```python
from build123d import *

# Parameters (mm, degrees)
EXTRUDE_1_DEPTH          = 2.5
SKETCH_4_W               = 70.612
SKETCH_4_H               = 2
EXTRUDE_2_DEPTH          = 10
SKETCH_5_R               = 4.19
SKETCH_5_R_2             = 4.191
EXTRUDE_3_DEPTH          = 12.5
SKETCH_7_R               = 2.7083489
SKETCH_7_R_2             = 2.708349387
CUT_EXTRUDE_1_DEPTH      = 10.5
CUT_EXTRUDE_2_DEPTH      = 48.585689944
CUT_EXTRUDE_2_DEPTH_BACK = 48.585689944
SKETCH_8_R               = 1.65


with BuildPart() as part:
    # 草图3 → 凸台-拉伸1 (new body)
    with BuildSketch(Plane.XY):
        with BuildLine():
            Line((-36.295196216, 26.676238556), (32.166947784, 26.676238556))
            ThreePointArc((32.166947784, 26.676238556), (32.927036662, 26.361399434), (33.241875784, 25.601310556))
            Line((33.241875784, 25.601310556), (33.241875784, -11.394297444))
            Line((33.241875784, -11.394297444), (-37.370124216, -11.320561244))
            Line((-37.370124216, -11.320561244), (-37.370124216, 25.601297856))
            ThreePointArc((-37.370124216, 25.601297856), (-37.055289584, 26.361394944), (-36.295196216, 26.676238556))
        make_face()
    extrude(amount=-EXTRUDE_1_DEPTH)

    # 草图4 → 凸台-拉伸2 (add)
    with BuildSketch(Plane(origin=(0, 0, -2.5), x_dir=(-1, 0, 0), z_dir=(0, 0, -1))):
        with Locations((2.064124216, -10.394297444)):
            Rectangle(SKETCH_4_W, SKETCH_4_H)
    extrude(amount=EXTRUDE_2_DEPTH)

    # 草图5 → 凸台-拉伸3 (add)
    with BuildSketch(Plane.XY):
        with Locations((-7.906124216, -5.962761444)):
            Circle(SKETCH_5_R)
        with Locations((28.796875784, 22.485238556)):
            Circle(SKETCH_5_R_2)
    extrude(amount=-EXTRUDE_3_DEPTH)

    # 草图7 → 切除-拉伸1 (cut)
    with BuildSketch(Plane.XY):
        with Locations((-7.906124216, -5.962761444)):
            Circle(SKETCH_7_R)
        with Locations((28.796875784, 22.485238556)):
            Circle(SKETCH_7_R_2)
    extrude(amount=-CUT_EXTRUDE_1_DEPTH, mode=Mode.SUBTRACT)

    # 草图8 → 切除-拉伸2 (cut, two sides: drawn at the far end of the back side and taken through both)
    with BuildSketch(Plane(origin=(0, 0, -12.5), x_dir=(-1, 0, 0), z_dir=(0, 0, -1)).offset(-CUT_EXTRUDE_2_DEPTH_BACK)):
        with Locations(Location((-28.796875784, 22.485238556, 0), (0, 0, 180))):
            Circle(SKETCH_8_R)
        with Locations(Location((7.906124216, -5.962761444, 0), (0, 0, 180))):
            Circle(SKETCH_8_R)
    extrude(amount=CUT_EXTRUDE_2_DEPTH + CUT_EXTRUDE_2_DEPTH_BACK, mode=Mode.SUBTRACT)


solid = part.part
```
The model under review builds one solid part; all positions refer to its coordinate system, in mm. A direction names the side the tool comes from. Round coordinates to 2 decimals unless told otherwise and drop trailing zeros. Write each loop counter-clockwise with the first axis right and the second up, starting at its lowest first coordinate (ties: lowest second). Pieces come first, ordered by that corner, then holes. Notation, with made-up numbers: M -33.75,69.5 L -12.75,69.5 A13 ccw -12.75,91.5 Z; hole C 80,62 d3. An arc over 180 degrees is marked long. Use CSV: the item, a comma, the result in double quotes. Start each with the question number.
(1) We need section A-A, the plane z = -9. State the section outline as (x, y) points, then the cut area to 3 significant figures.
(2) The part is to be moulded in two halves that separate along Y. For faces 4 (the face through (-37.37, 3, -2)), 5 (the face through (-3, 26.676, -1)), 6 (the face through (32.794, 23.744, -7.43)), say which applies: +Y half, -Y half, draft (parallel to the pull), parting line (faces both ways), or undercut.
(3) Clearance check with flat-ended pins moving along their axes: P1, Ø3, axis at y = -1.5, z = -7.5, coming from the +X side; P2, Ø4.5, axis at x = -7.91, y = -5.96, coming from the +Z side; P3, Ø3, axis at x = 4.5, z = -6.5, coming from the +Y side. State where each tip first meets the part, or that it passes through.
(4) We need section B-B, the plane y = -5. State the section outline as (x, z) points, then the cut area to 3 significant figures.
(5) We need section D-D, the plane y = 13. State the section outline as (x, z) points, then the cut area to 3 significant figures.
(6) Tool access review of faces 1 (the face through (14, -9.394, -7)), 2 (the face through (-2, 8, 0)), 3 (the face through (31.38, 23.3, -5.18)): name each direction out of +Z, -Z, +X, -X, +Y, -Y from which nothing blocks a thin tool from reaching the whole face with its end or side.
(7) For line 1 along Y through (x, z) = (28.5, -4.5); line 2 along Z through (x, y) = (-31, 4); line 3 along Y through (x, z) = (-27, -4.25), list the stretches that pass through material, from the lowest coordinate up.
Findings:
1,outline,"M -37.37,-11.39 L 33.24,-11.39 L 33.24,-9.39 L -5.5,-9.39 A4.19 ccw long -10.31,-9.39 L -37.37,-9.39 Z; C 28.8,22.49 d8.38; hole C -7.91,-5.96 d5.42; hole C 28.8,22.49 d5.42"
1,area,"203 mm^2"
2,face 4,"draft"
2,face 5,"+Y half"
2,face 6,"undercut"
3,P1,"x = -4.94"
3,P2,"z = -10.5"
3,P3,"y = -9.39"
4,outline,"M -37.37,-2.5 L -11.98,-2.5 L -11.98,-12.5 L -9.25,-12.5 L -9.25,-10.5 L -10.44,-10.5 L -10.44,0 L -37.37,0 Z; M -6.57,-12.5 L -3.83,-12.5 L -3.83,-2.5 L 33.24,-2.5 L 33.24,0 L -5.37,0 L -5.37,-10.5 L -6.57,-10.5 Z"
4,area,"200 mm^2"
5,outline,"M -37.37,-2.5 L 33.24,-2.5 L 33.24,0 L -37.37,0 Z"
5,area,"177 mm^2"
6,face 1,"-Z, +X"
6,face 2,"+Z, +X, -X, +Y, -Y"
6,face 3,"+Z"
7,line 1,"-11.39 to -9.39, 18.3 to 19.79, 25.18 to 26.67"
7,line 2,"-2.5 to 0"
7,line 3,"-11.39 to -9.39"
